Autodesk Inventor part; units mm, degrees
ref_plane "YZ Plane" through (0, 0, 0) normal (1, 0, 0) x (0, 1, 0)
ref_plane "XZ Plane" through (0, 0, 0) normal (0, 1, 0) x (-1, 0, 0)
ref_plane "XY Plane" through (0, 0, 0) normal (0, 0, 1) x (1, 0, 0)
sketch "Sketch1" plane through (0, 0, 0) normal (0, 0, 1) x (1, 0, 0)
  line L0 (0, 0) -> (0, 21.042)
  line L1 (0, 21.042) -> (29.758, 50.8)
  line L2 (29.758, 50.8) -> (50.8, 50.8)
  line L3 (50.8, 50.8) -> (50.8, 0)
  line L4 (50.8, 0) -> (0, 0)
  dimension "d0" = 50.8
  dimension "d2" = 50.8
  dimension "d3" = 50.8
  dimension "d4" = 135
extrude "Extrusion1" add sketch "Sketch1" along normal blind 3.175
sketch "Sketch2" plane through (0, 0, 3.175) normal (0, 0, 1) x (1, 0, 0)
  line L0 (50.8, 0) -> (50.8, 50.8)
  line L1 (0, 0) -> (50.8, 0)
  line L2 (50.8, 50.8) -> (47.625, 50.8)
  line L3 (47.625, 50.8) -> (47.625, 0)
  line L4 (47.625, 0) -> (50.8, 0)
  line L5 (50.8, 0) -> (50.8, 50.8)
  dimension "d7" = 3.175
extrude "Extrusion2" add sketch "Sketch2" against normal blind 50.8
sketch "Sketch3" plane through (50.8, 0, 3.175) normal (1, 0, 0) x (0, 0, -1)
  circle A0 centre (38.1, 13.8938) radius 3.3734
  circle A1 centre (12.7, 13.8938) radius 3.3734
  line L0 (0, 50.8) -> (50.8, 50.8)
  line L1 (0, 0) -> (0, 50.8)
  line L2 (0, 0) -> (50.8, 0)
  point P0 (3.175, 0)
  dimension "d10" = 6.7469
  dimension "d11" = 6.7469
  dimension "d14" = 12.7
  dimension "d15" = 25.4
  dimension "d25" = 13.8938
  dimension "d26" = 13.8938
extrude "Extrusion3" cut sketch "Sketch3" against normal blind 3.175
sketch "Sketch5" plane through (0, 0, 0) normal (0, 0, -1) x (-1, 0, 0)
  circle A0 centre (-11.7974, 14.879) radius 3.3734
  circle A1 centre (-29.758, 32.8395) radius 3.3734
  line L0 (0, 21.042) -> (-29.758, 50.8)
  line L1 (-29.758, 50.8) -> (-47.7185, 32.8395) construction
  point P0 (0, 0)
  dimension "d27" = 6.7469
  dimension "d28" = 6.7469
  dimension "d29" = 12.7
  dimension "d30" = 12.7
  dimension "d31" = 25.4
  dimension "d32" = 25.4
  dimension "d33" = 12.7
extrude "Extrusion5" cut sketch "Sketch5" against normal blind 3.175
properties part number "bottom left rail gusset" material "Aluminum 6061"
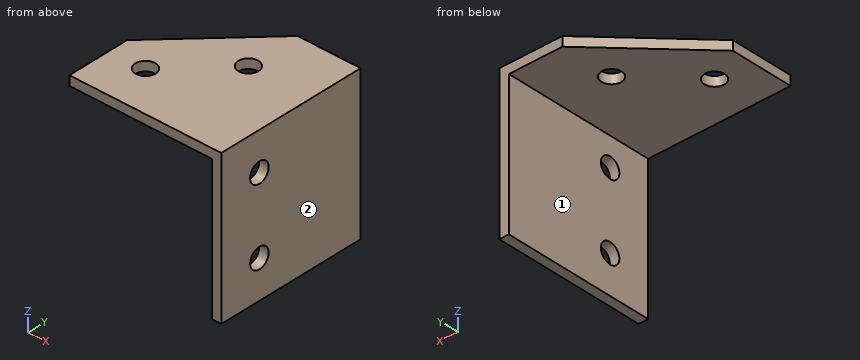
Verification items for the finished model (mm, model axes). Face numbers are marked on the shaded views. A direction names the side the tool comes from. Give positions to 0.01 mm unless a question says otherwise; leave off trailing zeros. Order: outer loops, then holes, each group sorted by start corner. A loop starts at its lowest first (then second) coordinate and runs counter-clockwise, first axis right, second up. Notation, with made-up numbers: M 10,-38 L 47,-38 A33 cw 47,0 Z; hole C -30,-26.5 d6. An arc over 180 degrees is marked long. Answer as a JSON object with one key per item and string values. Group by question number.
1) Depth check by flat-ended pin: pin 1 Ø8 at (x, y) = (11.8, 14.88) entering from -Z; pin 2 Ø1.5 at (y, z) = (38, -10.5) entering from -X (3 decimals). Enter the tip coordinate at first touch or a pass-through.
2) Cross-section at B-B (x = 31). Enter the section's corners in (y, z) (3 decimals).
3) Cross-section at A-A (y = 16.5). Enter the section's corners in (x, z) (3 decimals), then the cut area to 3 significant figures.
4) Cross-section at C-C (z = -8.5). Enter the section's corners in (x, y) (3 decimals), then the cut area to 3 significant figures.
5) Scan lines: line 1 along X through (y, z) = (16.5, -19) (3 decimals); line 2 along Z through (x, y) = (40.5, 34) (3 decimals); line 3 along X through (y, z) = (31.5, 1). Record each from-to range of solid material in increasing order. Write a range as [from, to].
6) Access from +Z, -Z, +X, -X, +Y, -Y to the whole of each face (thin tool, end or side, straight path). Record for the marked faces 1 and 2.
7) Cross-section at D-D (z = -28). Enter the section's corners in (x, y) (3 decimals), then the cut area to 3 significant figures.
Result sheet:
{
 "1": {"pin 1": "stops at z = 0", "pin 2": "stops at x = 47.625"},
 "2": {"outline": "M 0,0 L 29.703,0 L 29.703,3.175 L 0,3.175 Z; M 35.976,0 L 50.8,0 L 50.8,3.175 L 35.976,3.175 Z"},
 "3": {"outline": "M 0,0 L 8.839,0 L 8.839,3.175 L 0,3.175 Z; M 14.756,0 L 47.625,0 L 47.625,-7.383 L 50.8,-7.383 L 50.8,3.175 L 14.756,3.175 Z; M 47.625,-47.625 L 50.8,-47.625 L 50.8,-37.067 L 47.625,-37.067 Z; M 47.625,-32.783 L 50.8,-32.783 L 50.8,-11.667 L 47.625,-11.667 Z", "area": "267 mm2"},
 "4": {"outline": "M 47.625,0 L 50.8,0 L 50.8,10.68 L 47.625,10.68 Z; M 47.625,17.108 L 50.8,17.108 L 50.8,50.8 L 47.625,50.8 Z", "area": "141 mm2"},
 "5": {"line 1": "x = [47.625, 50.8]", "line 2": "z = [0, 3.175]", "line 3": "x = [10.46, 26.66], [32.85, 50.8]"},
 "6": {"face 1": "-Z, -X, +Y, -Y", "face 2": "+Z, -Z, +X, +Y, -Y"},
 "7": {"outline": "M 47.625,0 L 50.8,0 L 50.8,50.8 L 47.625,50.8 Z", "area": "161 mm2"}
}
